```python
from build123d import *

# Parameters (mm, degrees)
F0_W     = 100
F0_H     = 100
F1_DEPTH = 50
F2_R     = 40
F3_DEPTH = 50
F4_R     = 20
F5_DEPTH = 50


with BuildPart() as f1:
    # F0 (on Top) → F1 (new body)
    with BuildSketch(Plane.XY):
        with Locations((50, 50)):
            Rectangle(F0_W, F0_H)
    extrude(amount=F1_DEPTH)

    # F2 (on face) → F3 (join)
    with BuildSketch(Plane.XY.offset(50)):
        with Locations((50, 50)):
            Circle(F2_R)
    extrude(amount=F3_DEPTH)

    # F4 (on face) → F5 (join)
    with BuildSketch(Plane.XY.offset(100)):
        with Locations((50, 50)):
            Circle(F4_R)
    extrude(amount=F5_DEPTH)


solid = f1.part
```
The model under review builds one solid part; all positions refer to its coordinate system, in mm. A direction names the side the tool comes from. Give positions to 0.01 mm unless a question says otherwise; leave off trailing zeros. Write each loop counter-clockwise with the first axis right and the second up, starting at its lowest first coordinate (ties: lowest second). Pieces come first, ordered by that corner, then holes. Notation, with made-up numbers: M 9,22 L 59,22 A24 ccw 59,38 Z; hole C 40,33.25 d5. An arc over 180 degrees is marked long. Answer in a Markdown table with one row per item.
Item 1: Add section C-C on z = 91. Give the boundary of the cut face in (x, y), plus the area to 3 significant figures.
Check sheet entries:
| item | result |
|---|---|
| outline | C 50,50 d80 |
| area | 5,030 mm2 |
Item 2: Tool access review of faces 1 (the face through (0, 49, 25)), 2 (the face through (69.076, 56.007, 124.65)): name each direction out of +Z, -Z, +X, -X, +Y, -Y from which nothing blocks a thin tool from reaching the whole face with its end or side.
Check sheet entries:
| item | result |
|---|---|
| face 1 | +Z, -Z, -X, +Y, -Y |
| face 2 | +Z |
Item 3: For line 1 along Z through (x, y) = (55.5, 84); line 2 along Y through (x, z) = (50.5, 124.5); line 3 along Z through (x, y) = (92.5, 52), list the stretches that pass through material, from the lowest coordinate up.
Check sheet entries:
| item | result |
|---|---|
| line 1 | 0 to 100 |
| line 2 | 30.01 to 69.99 |
| line 3 | 0 to 50 |
Item 4: Add section D-D on y = 18. Give the boundary of the cut face in (x, z).
Check sheet entries:
| item | result |
|---|---|
| outline | M 0,0 L 100,0 L 100,50 L 74,50 L 74,100 L 26,100 L 26,50 L 0,50 Z |
Item 5: Add section A-A on y = 50. Give the boundary of the cut face in (x, z), plus the area to 3 significant figures.
Check sheet entries:
| item | result |
|---|---|
| outline | M 0,0 L 100,0 L 100,50 L 90,50 L 90,100 L 70,100 L 70,150 L 30,150 L 30,100 L 10,100 L 10,50 L 0,50 Z |
| area | 11,000 mm2 |
Item 6: For P1, Ø4, axis at x = 51, z = 74.5, coming from the -Y side; P2, Ø12, axis at x = 84.5, y = 87.5, coming from the +Z side; P3, Ø8, axis at y = 13.5, z = 62, coming from the +X side, all flat-tipped, find the tip position at first contact; note any pin that passes through.
Check sheet entries:
| item | result |
|---|---|
| P1 | y = 10 |
| P2 | z = 50 |
| P3 | x = 73.32 |
